Part model, mm, in its own coordinate system. A direction names the side the tool comes from. Coordinates: 2 decimals unless noted, no trailing zeros. Order: outer loops, then holes, each group sorted by start corner. A loop starts at its lowest first (then second) coordinate and runs counter-clockwise, first axis right, second up.
1) Tool access for faces 1 (the flat face through (-6, -44.5, -5)), 2 (the cylindrical face through (23.846, -0.623, 7.509)), 3 (the cylindrical face through (1.658, 49.43, -7.468)): list every direction of +Z, -Z, +X, -X, +Y, -Y with a clear straight run to the whole face (end or side of a thin tool).
2) Cut at D-D (z = 10). List the corners of the cut face in (x, y).
3) Cut at A-A (x = 0). List the corners of the cut face in (y, z), and give its area (3 significant figures).
4) Cut at C-C (y = -0.5). List the corners of the cut face in (x, z).
5) Wall check: L1, parallel to Y at x = -3.5, z = 20; L2, parallel to X at y = -9.5, z = -9; L3, parallel to Z at x = -5, y = -16. Give the ranges that are in metal, low to high.
6) Pin check, flat tips, straight feed: pin 1 Ø8 at (x, z) = (19.5, -19.5) entering from -Y; pin 2 Ø5 at (x, y) = (6.5, -18) entering from +Z; pin 3 Ø6 at (y, z) = (43.5, -7) entering from -X. Stop position of each tip, or through.
7) Cut at B-B (z = 0). List the corners of the cut face in (x, y).
```python
from build123d import *

# Parameters (mm, degrees)
F0_R     = 25
F1_DEPTH = 44.5
F2_R     = 7.65
F3_DEPTH = 10
F4_R     = 7.65
F5_DEPTH = 10


with BuildPart() as f1:
    # F0 (on Front) → F1 (new body, symmetric)
    with BuildSketch(Plane.XZ):
        Circle(F0_R)
    extrude(amount=F1_DEPTH, both=True)

    # F2 (on face) → F3 (join)
    with BuildSketch(Plane(origin=(0, 44.5, 0), x_dir=(-1, 0, 0), z_dir=(0, 1, 0))):
        Circle(F2_R)
    extrude(amount=F3_DEPTH)

    # F4 (on face) → F5 (join)
    with BuildSketch(Plane.XZ.offset(44.5)):
        Circle(F4_R)
    extrude(amount=F5_DEPTH)


solid = f1.part
```
Geometry check:
1. face 1: -Y
1. face 2: +Y, -Y
1. face 3: +Y
2. outline: (-22.91, -44.5) - (22.91, -44.5) - (22.91, 44.5) - (-22.91, 44.5) - close
3. outline: (-54.5, -7.65) - (-44.5, -7.65) - (-44.5, -25) - (44.5, -25) - (44.5, -7.65) - (54.5, -7.65) - (54.5, 7.65) - (44.5, 7.65) - (44.5, 25) - (-44.5, 25) - (-44.5, 7.65) - (-54.5, 7.65) - close
3. area: 4,760 mm2
4. outline: circle Ø50 at (0, 0)
5. L1: y = -44.5 to 44.5
5. L2: x = -23.32 to 23.32
5. L3: z = -24.49 to 24.49
6. pin 1: stops at y = -44.5
6. pin 2: stops at z = 24.68
6. pin 3: stops at x = -24.68
7. outline: (-25, -44.5) - (-7.65, -44.5) - (-7.65, -54.5) - (7.65, -54.5) - (7.65, -44.5) - (25, -44.5) - (25, 44.5) - (7.65, 44.5) - (7.65, 54.5) - (-7.65, 54.5) - (-7.65, 44.5) - (-25, 44.5) - close
